from build123d import *

# Parameters (mm, degrees)
SKETCH1_W             = 15.5
SKETCH1_H             = 62
BOSS_EXTRUDE1_DEPTH   = 62
FILLET1_R             = 3
CUT_EXTRUDE1_REACH    = 71.958
CUT_EXTRUDE2_DEPTH    = 42
FILLET2_R             = 5
M6_TAPPED_HOLE1_D     = 5
M6_TAPPED_HOLE1_DEPTH = 15
M6_TAPPED_HOLE1_TIP   = 1.502151548


with BuildPart() as part:
    # Sketch1 → Boss-Extrude1 (new body)
    with BuildSketch(Plane(origin=(0, 0, 0), x_dir=(1, 0, 0), z_dir=(0, 1, 0))):
        with Locations((-0.38, -0.37)):
            Rectangle(SKETCH1_W, SKETCH1_H)
    extrude(amount=-BOSS_EXTRUDE1_DEPTH)

    # Fillet1
    fillet1_edges = [part.edges().sort_by_distance(p)[0] for p in [
        (7.37, -31, 31.37),
        (-8.13, -31, 31.37),
        (-8.13, -31, -30.63),
        (7.37, -31, -30.63),
    ]]
    fillet(fillet1_edges, radius=FILLET1_R)

    # Sketch2 → Cut-Extrude1 (cut, up to next)
    with BuildSketch(Plane(origin=(0, 0, 0), x_dir=(1, 0, 0), z_dir=(0, 1, 0)), mode=Mode.PRIVATE) as cut_extrude1_sk1:
        with BuildLine():
            Line((-5.13, 10.63), (0.37, 10.63))
            ThreePointArc((0.37, 10.63), (1.784213562, 10.044213562), (2.37, 8.63))
            Line((2.37, 8.63), (2.37, -9.37))
            ThreePointArc((2.37, -9.37), (1.784213562, -10.784213562), (0.37, -11.37))
            Line((0.37, -11.37), (-5.13, -11.37))
            ThreePointArc((-5.13, -11.37), (-7.251320344, -12.248679656), (-8.13, -14.37))
            Line((-8.13, -14.37), (-8.13, 13.63))
            ThreePointArc((-8.13, 13.63), (-7.251320344, 11.508679656), (-5.13, 10.63))
        make_face()
    cut_extrude1_tool1 = extrude(cut_extrude1_sk1.sketch, amount=-CUT_EXTRUDE1_REACH, mode=Mode.PRIVATE) & part.part
    add(cut_extrude1_tool1.solids().sort_by_distance((-2.991251, 0, 0.37))[0], mode=Mode.SUBTRACT)

    # Sketch3 → Cut-Extrude2 (cut)
    with BuildSketch(Plane(origin=(0, -62, 0), x_dir=(1, 0, 0), z_dir=(0, 1, 0))):
        with BuildLine():
            Line((4.37, -16.37), (-8.13, -16.37))
            Line((-8.13, -16.37), (-8.13, -28.37))
            ThreePointArc((-8.13, -28.37), (-7.251320344, -30.491320344), (-5.13, -31.37))
            Line((-5.13, -31.37), (4.37, -31.37))
            ThreePointArc((4.37, -31.37), (6.491320344, -30.491320344), (7.37, -28.37))
            Line((7.37, -28.37), (7.37, -13.37))
            ThreePointArc((7.37, -13.37), (6.491320344, -15.491320344), (4.37, -16.37))
        make_face()
    cut_extrude2 = extrude(amount=CUT_EXTRUDE2_DEPTH, mode=Mode.SUBTRACT)

    # Mirror1: Cut-Extrude2 across plane
    add(cut_extrude2.mirror(Plane.XY), mode=Mode.SUBTRACT)

    # Fillet2
    # the kernel refuses this fillet: 5 mm, written as the material it adds along each edge
    with BuildSketch(Plane(origin=(4.37, -20, -16.37), x_dir=(0, -1, 0), z_dir=(-1, 0, 0)), Plane(origin=(4.37, -20, 16.37), x_dir=(0, 0, 1), z_dir=(-1, 0, 0))) as fillet2_piece_1:
        with BuildLine():
            CenterArc((FILLET2_R, -FILLET2_R), FILLET2_R, 90, 90)
            Line((0, -FILLET2_R), (0, 0))
            Line((0, 0), (FILLET2_R, 0))
        make_face()
    extrude(amount=12.5)
    with BuildSketch(Plane(origin=(4.37, -20, -13.37), x_dir=(-0.5176042277799098, 0, -0.855620163030514), z_dir=(0.855620163030514, 0, -0.5176042277799098))) as fillet2_piece_2_section:
        with BuildLine():
            CenterArc((-3 - FILLET2_R, -FILLET2_R), FILLET2_R, 0, 90)
            Line((-3, -FILLET2_R), (-3, 0))
            Line((-3, 0), (-3 - FILLET2_R, 0))
        make_face()
    fillet2_piece_2 = revolve(axis=Axis((4.37, -20, -13.37), (0, 1, 0)), revolution_arc=328.828315396, mode=Mode.PRIVATE)
    fillet2_piece_2 = split(fillet2_piece_2, bisect_by=Plane(origin=(6.644254363, -21.721658314, -10.63), z_dir=(0, 0, -1)), keep=Keep.TOP, mode=Mode.PRIVATE)
    fillet2_piece_2 = split(fillet2_piece_2, bisect_by=Plane(origin=(7.37, -21.721658314, -15.644254458), z_dir=(-1, 0, 0)), keep=Keep.TOP, mode=Mode.PRIVATE)
    add(fillet2_piece_2)
    with BuildSketch(Plane(origin=(4.37, -20, 13.37), x_dir=(-0.5176042277799098, 0, 0.855620163030514), z_dir=(0.855620163030514, 0, 0.5176042277799098))) as fillet2_piece_3_section:
        with BuildLine():
            CenterArc((-3 - FILLET2_R, FILLET2_R), FILLET2_R, 270, 90)
            Line((-3, FILLET2_R), (-3, 0))
            Line((-3, 0), (-3 - FILLET2_R, 0))
        make_face()
    fillet2_piece_3 = revolve(axis=Axis((4.37, -20, 13.37), (0, -1, 0)), revolution_arc=328.828315396, mode=Mode.PRIVATE)
    fillet2_piece_3 = split(fillet2_piece_3, bisect_by=Plane(origin=(6.644254403, -21.721658525, 11.37), z_dir=(0, 0, 1)), keep=Keep.TOP, mode=Mode.PRIVATE)
    fillet2_piece_3 = split(fillet2_piece_3, bisect_by=Plane(origin=(7.37, -21.721658525, 15.644254403), z_dir=(-1, 0, 0)), keep=Keep.TOP, mode=Mode.PRIVATE)
    add(fillet2_piece_3)

    # M6 Tapped Hole1
    with Locations(Plane(origin=(0, 0, 0), x_dir=(1, 0, 0), z_dir=(0, 1, 0))):
        with Locations((-0.38, 20.63), (-0.38, -21.37)):
            Hole(M6_TAPPED_HOLE1_D / 2, depth=M6_TAPPED_HOLE1_DEPTH)
            with Locations((0, 0, -(M6_TAPPED_HOLE1_DEPTH + M6_TAPPED_HOLE1_TIP / 2))):  # 118° drill point
                Cone(0, M6_TAPPED_HOLE1_D / 2, M6_TAPPED_HOLE1_TIP, mode=Mode.SUBTRACT)


solid = part.part
Work out the finished part from the listing and answer in its coordinate system (mm). A direction names the side the tool comes from. Round coordinates to 2 decimals unless told otherwise and drop trailing zeros. Write each loop counter-clockwise with the first axis right and the second up, starting at its lowest first coordinate (ties: lowest second). Pieces come first, ordered by that corner, then holes.
1) Straight lines are drawn through the part: line 1 (Z direction, x = -0.38, y = -9.5); line 2 (X direction, y = -6.5, z = -20.63); line 3 (Z direction, x = 0.25, y = -45). For each, find the intervals that lie inside material, in ascending order.
2) A cutting plane is placed at A-A (x = -4). Give the vertices of the cut face in (y, z).
3) The mould has two halves that part along Z. Classify faces 4 (the cylindrical face through (1.77, -30.57, -10.06)), 5 (the cylindrical face through (-7.3, -10.1, -29.7)), 6 (the flat face through (0, -10, 31.37)): pulls with the +Z half, pulls with the -Z half, needs draft (parallel to the pull), parting line crosses it, or undercut.
4) A cutting plane is placed at B-B (y = -53). Give the vertices of the cut face in (x, z).
5) Given pin 1 Ø4 at (x, z) = (-0.38, 21.37) entering from +Y; pin 2 Ø2 at (y, z) = (-17.5, -2.5) entering from -X; pin 3 Ø4.5 at (x, y) = (-2, -33) entering from -Z, each flat-ended and moving along its own axis, determine where each tip first touches the part or whether it passes through.
6) A tool of negligible diameter and unlimited length cuts with its end or side. For faces 1 (the cylindrical face through (1.8, -30.57, 10.77)), 2 (the flat face through (0, -20, 26)), 3 (the flat face through (-2, -44, -16.37)), from which of +Z, -Z, +X, -X, +Y, -Y can it reach the whole face along a straight path? Write none if from no direction.
7) A cutting plane is placed at C-C (z = 25.5). Give the vertices of the cut face in (x, y), plus the area to 3 significant figures.
Completed:
1. line 1: z = -30.63 to -23.13, -18.13 to -10.63, 11.37 to 18.87, 23.87 to 31.37
1. line 2: x = -8.13 to -2.88, 2.12 to 7.37
1. line 3: z = -16.37 to -10.63, 11.37 to 16.37
2. outline: (-62, -16.37) - (-25, -16.37) arc R5 cw to (-20, -21.37) - (-20, -30.63) - (0, -30.63) - (0, -10.63) - (-62, -10.63) - close; (-62, 11.37) - (0, 11.37) - (0, 31.37) - (-20, 31.37) - (-20, 21.37) arc R5 cw to (-25, 16.37) - (-62, 16.37) - close
3. face 4: undercut
3. face 5: pulls with the -Z half
3. face 6: pulls with the +Z half
4. outline: (-8.13, -16.37) - (4.37, -16.37) arc R3 ccw to (7.37, -13.37) - (7.37, 13.37) arc R3 ccw to (4.37, 16.37) - (-8.13, 16.37) - (-8.13, 14.37) arc R3 ccw to (-5.13, 11.37) - (0.37, 11.37) arc R2 cw to (2.37, 9.37) - (2.37, -8.63) arc R2 cw to (0.37, -10.63) - (-5.13, -10.63) arc R3 ccw to (-8.13, -13.63) - close
5. pin 1: stops at y = -15.3
5. pin 2: stops at x = 2.37
5. pin 3: stops at z = -16.37
6. face 1: -X, +Y, -Y
6. face 2: +Z, +X, -X, -Y
6. face 3: -Z, +X, -X, -Y
7. outline: (-8.13, -20) - (7.37, -20) - (7.37, 0) - (-8.13, 0) - close
7. area: 310 mm2
